from build123d import *
from build123d.topology import SkipClean

# Parameters (mm, degrees)
SKETCH1_R           = 10
BOSS_EXTRUDE1_DEPTH = 10
SKETCH4_R           = 1.305
CUT_EXTRUDE3_DEPTH  = 25.5
BOSS_EXTRUDE2_START = 4.5
BOSS_EXTRUDE2_DEPTH = 4.5
SKETCH6_R           = 0.935
CUT_EXTRUDE4_DEPTH  = 12.25
SKETCH7_W           = 11.364916732
SKETCH7_H           = 5
BOSS_EXTRUDE3_DEPTH = 4.5
SKETCH8_R           = 0.935
CUT_EXTRUDE5_DEPTH  = 7.25
BOSS_EXTRUDE4_DEPTH = 4.5
CUT_EXTRUDE6_START  = -0.75
CUT_EXTRUDE6_DEPTH  = 0.75
SKETCH12_W          = 5.25
SKETCH12_H          = 4
CUT_EXTRUDE7_DEPTH  = 1.6
CUT_EXTRUDE8_DEPTH  = 15.8
FILLET1_R           = 2
CUT_EXTRUDE9_DEPTH  = 10.8
SKETCH15_W          = 11.364916732
SKETCH15_H          = 6.6
CUT_EXTRUDE10_DEPTH = 1.6
CUT_EXTRUDE11_DEPTH = 15
BOSS_EXTRUDE5_REACH = 35.438
SKETCH17_R          = 10
SKETCH17_R_2        = 1.305
CUT_EXTRUDE12_DEPTH = 14
SCALE1_SCALE        = 0.8


# Read off the part's stored shape, not the designer's step: Cut-Extrude6
with BuildPart() as part:
    # Sketch1 → Boss-Extrude1 (new, symmetric)
    with BuildSketch(Plane(origin=(0, 0, 0), x_dir=(0, 0, -1), z_dir=(1, 0, 0))):
        Circle(SKETCH1_R)
    extrude(amount=BOSS_EXTRUDE1_DEPTH, both=True)

    # Sketch4 → Cut-Extrude3 (cut, symmetric)
    with BuildSketch(Plane(origin=(0, -0.76336978, 0), x_dir=(0, 0, -1), z_dir=(1, 0, 0))):
        with Locations((0, -6.913267104)):
            Circle(SKETCH4_R)
    extrude(amount=CUT_EXTRUDE3_DEPTH, both=True, mode=Mode.SUBTRACT)

    # Sketch5 → Boss-Extrude2 (add)
    with BuildSketch(Plane(origin=(10, 0, 0), x_dir=(0, 0, -1), z_dir=(1, 0, 0)).offset(BOSS_EXTRUDE2_START)):
        with BuildLine():
            Line((-9.682458366, -2.5), (-5.682458366, -2.5))
            Line((-5.682458366, -2.5), (-5.682458366, 2.5))
            Line((-5.682458366, 2.5), (-9.682458366, 2.5))
            ThreePointArc((-9.682458366, 2.5), (-10, 0), (-9.682458366, -2.5))
        make_face()
    boss_extrude2 = extrude(amount=-BOSS_EXTRUDE2_DEPTH)

    # Mirror1: Boss-Extrude2 across plane
    add(boss_extrude2.mirror(Plane.XY))

    # Sketch6 → Cut-Extrude4 (cut, symmetric)
    with SkipClean():  # the faces are left unmerged after this step: merging them gives an invalid solid
        with BuildSketch(Plane.XY):
            with Locations((12.25, 0.25)):
                Circle(SKETCH6_R)
        extrude(amount=CUT_EXTRUDE4_DEPTH, both=True, mode=Mode.SUBTRACT)

    # Sketch7 → Boss-Extrude3 (add)
    with SkipClean():  # the faces are left unmerged after this step: merging them gives an invalid solid
        with BuildSketch(Plane.ZY.offset(10)):
            Rectangle(SKETCH7_W, SKETCH7_H)
        extrude(amount=BOSS_EXTRUDE3_DEPTH)

    # Sketch8 → Cut-Extrude5 (cut, symmetric)
    with SkipClean():  # the faces are left unmerged after this step: merging them gives an invalid solid
        with BuildSketch(Plane.XY):
            with Locations((-12.25, 0.25)):
                Circle(SKETCH8_R)
        extrude(amount=CUT_EXTRUDE5_DEPTH, both=True, mode=Mode.SUBTRACT)

    # Sketch10 → Boss-Extrude4 (add)
    with SkipClean():  # the faces are left unmerged after this step: merging them gives an invalid solid
        with BuildSketch(Plane.ZY.offset(10)):
            with BuildLine():
                Line((9.682458366, 2.5), (-9.682458366, 2.5))
                ThreePointArc((-9.682458366, 2.5), (0, 10), (9.682458366, 2.5))
            make_face()
        extrude(amount=BOSS_EXTRUDE4_DEPTH)

    # Cut-Extrude6 outline → Cut-Extrude6 (cut)
    with SkipClean():  # the faces are left unmerged after this step: merging them gives an invalid solid
        with BuildSketch(Plane.ZY.offset(10).offset(CUT_EXTRUDE6_START)):
            with BuildLine():
                ThreePointArc((-9.682458366, 2.5), (-9.369942303, -3.493448331), (-5.682458366, -8.228588392))
                Line((-5.682458366, -8.228588392), (-5.682458366, 2.5))
                Line((-5.682458366, 2.5), (-9.682458366, 2.5))
            make_face()
            with BuildLine():
                Line((5.682458366, 2.5), (5.682458366, -8.228588392))
                ThreePointArc((5.682458366, -8.228588392), (9.369942303, -3.493448331), (9.682458366, 2.5))
                Line((9.682458366, 2.5), (5.682458366, 2.5))
            make_face()
        extrude(amount=CUT_EXTRUDE6_DEPTH, mode=Mode.SUBTRACT)

    # Sketch12 → Cut-Extrude7 (cut)
    with SkipClean():  # the faces are left unmerged after this step: merging them gives an invalid solid
        with BuildSketch(Plane.XZ.offset(-2.5)):
            with Locations((-11.875, -7.682458366)):
                Rectangle(SKETCH12_W, SKETCH12_H)
            with Locations((-11.875, 7.682458366)):
                Rectangle(SKETCH12_W, SKETCH12_H)
        extrude(amount=-CUT_EXTRUDE7_DEPTH, mode=Mode.SUBTRACT)

    # Sketch13 → Cut-Extrude8 (cut, symmetric)
    with SkipClean():  # the faces are left unmerged after this step: merging them gives an invalid solid
        with BuildSketch(Plane.XY):
            Polygon((-10, -8.228588392), (-10, -2.5), (-2.5, -10), (-10, -10), align=None)
        extrude(amount=CUT_EXTRUDE8_DEPTH, both=True, mode=Mode.SUBTRACT)

    # Fillet1
    fillet1_edges = [part.edges().sort_by_distance(p)[0] for p in [
        (14.5, -2.5, 7.682458366),
        (14.5, -2.5, -7.682458366),
    ]]
    fillet(fillet1_edges, radius=FILLET1_R)

    # Sketch14 → Cut-Extrude9 (cut, symmetric)
    with SkipClean():  # the faces are left unmerged after this step: merging them gives an invalid solid
        with BuildSketch(Plane.XY):
            Polygon((10, -10), (10, -2.5), (2.5, -10), align=None)
        extrude(amount=CUT_EXTRUDE9_DEPTH, both=True, mode=Mode.SUBTRACT)

    # Sketch15 → Cut-Extrude10 (cut)
    with SkipClean():  # the faces are left unmerged after this step: merging them gives an invalid solid
        with BuildSketch(Plane(origin=(10, 0, 0), x_dir=(0, 0, -1), z_dir=(1, 0, 0))):
            with Locations((0, -0.8)):
                Rectangle(SKETCH15_W, SKETCH15_H)
        extrude(amount=-CUT_EXTRUDE10_DEPTH, mode=Mode.SUBTRACT)

    # Sketch16 → Cut-Extrude11 (cut)
    with SkipClean():  # the faces are left unmerged after this step: merging them gives an invalid solid
        with BuildSketch(Plane(origin=(10, 0, 0), x_dir=(0, 0, -1), z_dir=(1, 0, 0))):
            with BuildLine():
                Line((-5.75, 5.5), (-5.75, -5.5))
                Line((-5.75, -5.5), (5.75, -5.5))
                Line((5.75, -5.5), (5.75, 5.5))
                ThreePointArc((5.75, 5.5), (0, 7.956915231), (-5.75, 5.5))
            make_face()
        extrude(amount=-CUT_EXTRUDE11_DEPTH, mode=Mode.SUBTRACT)


with BuildPart() as body_2:
    # Split1: the piece on the far side of the plane
    add(part.part)
    split(bisect_by=Plane(origin=(0, 0, 0), x_dir=(0, 0, 1), z_dir=(1, 0, 0)), keep=Keep.BOTTOM)


with BuildPart() as part_1:
    add(part.part)

    # Split1
    split(bisect_by=Plane(origin=(0, 0, 0), x_dir=(0, 0, 1), z_dir=(1, 0, 0)), keep=Keep.TOP)


with BuildPart() as part_2:
    # Body-Move/Copy1: moved
    add(part_1.part.moved(Location((15.8, 0, 0))))


    # Sketch17 → Boss-Extrude5 (add, up to next)
    with BuildSketch(Plane.ZY.offset(-15.8), mode=Mode.PRIVATE) as boss_extrude5_sk1:
        with Locations(Location((0, 0, 0), (0, 0, 357.134016017))):
            Circle(SKETCH17_R)
        with Locations(Location((0, -7.676636884, 0), (0, 0, 180))):
            Circle(SKETCH17_R_2, mode=Mode.SUBTRACT)
        with BuildLine():
            Line((-5.75, -5.5), (5.75, -5.5))
            Line((5.75, -5.5), (5.75, 5.5))
            ThreePointArc((5.75, 5.5), (0, 7.956915231), (-5.75, 5.5))
            Line((-5.75, 5.5), (-5.75, -5.5))
        make_face(mode=Mode.SUBTRACT)
    boss_extrude5_tool1 = extrude(boss_extrude5_sk1.sketch, amount=BOSS_EXTRUDE5_REACH, mode=Mode.PRIVATE) - body_2.part
    add(boss_extrude5_tool1.solids().sort_by_distance((15.8, 0.485858, -9.705003))[0])


with BuildPart() as body_2_1:
    # Body-Move/Copy2: moved
    add(body_2.part.moved(Location((9.26, 0, 0))))

    # Combine4: union part
    add(part_2.part)

    # Sketch18 → Cut-Extrude12 (cut)
    with SkipClean():  # the faces are left unmerged after this step: merging them gives an invalid solid
        with BuildSketch(Plane.ZY.offset(5.24)):
            with BuildLine():
                Line((-5.75, 5.5), (-5.75, 4.1))
                Line((-5.75, 4.1), (5.75, 4.1))
                Line((5.75, 4.1), (5.75, 5.5))
                ThreePointArc((5.75, 5.5), (0, 7.956915231), (-5.75, 5.5))
            make_face()
        extrude(amount=-CUT_EXTRUDE12_DEPTH, mode=Mode.SUBTRACT)


with BuildPart() as body_2_2:
    # Scale1: scaled about (10.157754057, 0.26372377, 1.86e-07)
    add(body_2_1.part.scale(SCALE1_SCALE).moved(Location((2.031550811, 0.052744754, 3.7e-08))))


solid = body_2_2.part
Model file for the job. Use its own axes, mm. A direction names the side the tool comes from. Round coordinates to 2 decimals unless told otherwise and drop trailing zeros. Loops run counter-clockwise (first coordinate to the right, second up) from the corner with the lowest first, then second, coordinate; pieces in that order, holes last.
1. Band-saw the part on C-C, the plane x = 16.25. List the corners of the cut face in (y, z).
Check values:
outline: circle Ø16 at (0.05, 0); hole circle Ø2.09 at (-6.09, 0); hole (-4.35, -4.6) - (4.45, -4.6) arc R6.37 ccw to (4.45, 4.6) - (-4.35, 4.6) - close
2. Band-saw the part on D-D, the plane y = 4. List the corners of the cut face in (x, z), and give its area (3 significant figures).
Check values:
outline: (-2.16, -6.96) - (22.67, -6.96) - (22.67, -4.6) - (-2.16, -4.6) - close; (-2.16, 4.6) - (22.67, 4.6) - (22.67, 6.96) - (-2.16, 6.96) - close
area: 117 mm2
3. Mould opens along Z. For faces 4 (the flat face through (23.7, -0.4, -4.546)), 5 (the flat face through (24, 2.053, 6)) say: +Z half, -Z half, draft (parallel to the pull), parting line (faces both ways), or undercut.
Check values:
face 4: undercut
face 5: draft
4. Wall check: probe 1 along X at (y, z) = (-1.25, 4.25); probe 2 along Z at (x, y) = (14.75, 2.25); probe 3 along X at (y, z) = (4.25, 6.5). Give the ranges that are in metal, low to high.
Check values:
probe 1: x = -2.16 to 5.44
probe 2: z = -7.69 to -4.6, 4.6 to 7.69
probe 3: x = -2.16 to 22.67
5. Drop flat-ended pins along their axis: P1, Ø2, axis at x = 10.5, z = -3.5, coming from the -Y side; P2, Ø1.5, axis at x = 11.5, y = 6, coming from the -Z side; P3, Ø1, axis at y = -5, z = -2, coming from the +X side. Give the stop position or say it passes through.
Check values:
P1: stops at y = -7.55
P2: stops at z = -6.08
P3: stops at x = 20.12
6. Tool access for faces 1 (the flat face through (2, 3.333, 0)), 2 (the flat face through (24, -1.947, -6)), 3 (the flat face through (0, 3.333, 6)): list every direction of +Z, -Z, +X, -X, +Y, -Y with a clear straight run to the whole face (end or side of a thin tool).
Check values:
face 1: +X, -X
face 2: +Z, -Z, +X, -Y
face 3: +Z, -X, -Y
7. Band-saw the part on B-B, the plane z = 0. List the corners of the cut face in (x, y).
Check values:
outline: (-2.16, -1.95) - (1.44, -1.95) - (3.84, -4.35) - (2.03, -4.35) - (2.03, -5.04) - (19.57, -5.04) - (20.27, -4.35) - (5.44, -4.35) - (5.44, 3.33) - (-2.16, 3.33) - close; (-2.16, 6.42) - (22.67, 6.42) - (22.67, 8.05) - (-2.16, 8.05) - close; (2.03, -7.95) - (16.67, -7.95) - (17.49, -7.13) - (2.03, -7.13) - close; hole circle Ø1.5 at (-0.36, 0.25)
8. Band-saw the part on A-A, the plane z = 4.25. List the corners of the cut face in (x, y), and give its area (3 significant figures).
Check values:
outline: (-2.16, -1.95) - (1.44, -1.95) - (3.84, -4.35) - (2.03, -4.35) - (2.03, -6.72) - (17.89, -6.72) - (20.27, -4.35) - (5.44, -4.35) - (5.44, 3.33) - (-2.16, 3.33) - close; (-2.16, 4.79) - (22.67, 4.79) - (22.67, 6.83) - (-2.16, 6.83) - close; hole circle Ø1.5 at (-0.36, 0.25)
area: 136 mm2
